```python
from build123d import *

# Parameters (mm, degrees)
SKETCH_1_W                = 6
SKETCH_1_H                = 107
SKETCH_3_W                = 19.4
SKETCH_3_H                = 3
INTERNAL_OUTPUT_KEY_DEPTH = 5
SKETCH_4_R                = 4.3
SCREW_CLEARANCE_DEPTH     = 52


with BuildPart() as part:
    # 草图1 → Output_tube (revolve)
    with BuildSketch(Plane.XY, mode=Mode.PRIVATE) as output_tube_sk:
        with Locations((3, 53.5)):
            Rectangle(SKETCH_1_W, SKETCH_1_H)
    revolve(output_tube_sk.sketch.rotate(Axis((0, 0, 0), (0, 1, 0)), 90), axis=Axis((0, 0, 0), (0, 1, 0)))

    # 草图3 → Internal_output_key (add)
    with BuildSketch(Plane.XY.offset(-2.5)):
        with Locations((0, 104.5)):
            Rectangle(SKETCH_3_W, SKETCH_3_H)
    extrude(amount=INTERNAL_OUTPUT_KEY_DEPTH)

    # 草图4 → Screw_clearance (cut)
    with BuildSketch(Plane(origin=(0, 107, 0), x_dir=(1, 0, 0), z_dir=(0, 1, 0))):
        with Locations(Location((0, 0, 0), (0, 0, 270))):
            Circle(SKETCH_4_R)
    extrude(amount=-SCREW_CLEARANCE_DEPTH, mode=Mode.SUBTRACT)


solid = part.part
```
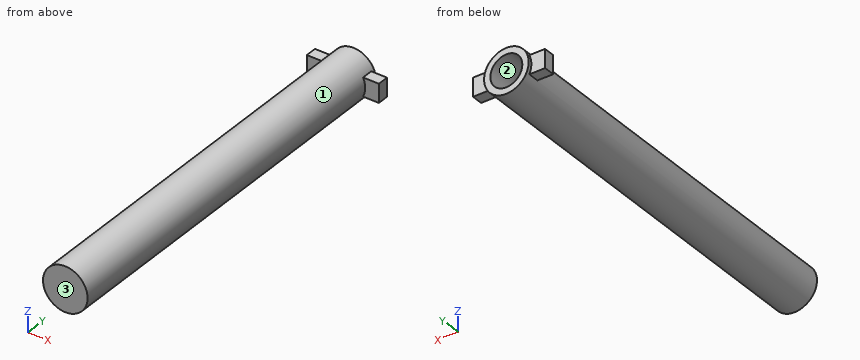
Could you check a few things on this model? Use its own coordinates, in mm. Face numbers are marked on the shaded views. Give positions to 0.01 mm unless a question says otherwise; leave off trailing zeros. Order: outer loops, then holes, each group sorted by start corner. A loop starts at its lowest first (then second) coordinate and runs counter-clockwise, first axis right, second up.
Q1. If I drill on line 1 along X through (y, z) = (90, 0); line 2 along Y through (x, z) = (7.75, 0.25); line 3 along Y through (x, z) = (1.75, 3), over which ranges is the centre line in solid material (lowest first)?
Q2. Suppose I cut it at B-B, the plane z = 0. Write out the boundary of the cut face in (x, y).
Q3. Suppose I cut it at A-A, the plane x = 0. Write out the boundary of the cut face in (y, z), and give its area (3 significant figures).
Q4. Suppose I cut it at C-C, the plane y = 56. Write out the boundary of the cut face in (x, z).
Q5. We'd pull the mould along Z, two halves only. Please class the marked faces 1, 2 and 3: +Z half, -Z half, draft (parallel to the pull), parting line (faces both ways), or undercut.
Q6. I'm going to push flat-ended pins straight in: P1, Ø2.5, axis at x = 7.5, y = 104.5, coming from the +Z side; P2, Ø1.5, axis at x = 1, y = 28, coming from the +Z side; P3, Ø6, axis at y = 71.5, z = -3, coming from the -X side. Where does each tip first touch, or does it pass through?
Solution:
1. line 1: x = -6 to -4.3, 4.3 to 6
1. line 2: y = 103 to 106
1. line 3: y = 0 to 55
2. outline: (-9.7, 103) - (-6, 103) - (-6, 0) - (6, 0) - (6, 103) - (9.7, 103) - (9.7, 106) - (6, 106) - (6, 107) - (4.3, 107) - (4.3, 55) - (-4.3, 55) - (-4.3, 107) - (-6, 107) - (-6, 106) - (-9.7, 106) - close
3. outline: (0, -6) - (107, -6) - (107, -4.3) - (55, -4.3) - (55, 4.3) - (107, 4.3) - (107, 6) - (0, 6) - close
3. area: 837 mm2
4. outline: circle Ø12 at (0, 0); hole circle Ø8.6 at (0, 0)
5. face 1: parting line
5. face 2: undercut
5. face 3: draft
6. P1: stops at z = 2.5
6. P2: stops at z = 5.99
6. P3: stops at x = -6
